```python
from build123d import *

# Parameters (mm, degrees)
SKETCH1_W           = 82.539998569
SKETCH1_H           = 65.04
BOSS_EXTRUDE1_DEPTH = 43.18
SHELL1_T            = 2.54
CUT_EXTRUDE2_DEPTH  = 124.028758627
SKETCH7_W           = 87.619998569
SKETCH7_H           = 43.18
BOSS_EXTRUDE2_DEPTH = 2.54
CUT_EXTRUDE3_DEPTH  = 2.54
CUT_EXTRUDE4_DEPTH  = 2.54
SKETCH10_W          = 1.27
SKETCH10_H          = 35.56
CUT_EXTRUDE5_DEPTH  = 2.54
SKETCH11_W          = 12.7
SKETCH11_H          = 2.54
BOSS_EXTRUDE3_DEPTH = 12.7
CUT_EXTRUDE7_DEPTH  = 125.717897357
SKETCH13_W          = 12.7
SKETCH13_H          = 12.7
SKETCH13_R          = 2.1
BOSS_EXTRUDE4_DEPTH = 3.175
FILLET2_R           = 3


with BuildPart() as part:
    # Sketch1 → Boss-Extrude1 (new body)
    with BuildSketch(Plane.XY):
        with Locations((47.599999189, 40.75)):
            Rectangle(SKETCH1_W, SKETCH1_H)
    extrude(amount=BOSS_EXTRUDE1_DEPTH)

    # Shell1
    shell1_openings = [part.faces().sort_by_distance(p)[0] for p in [
        (47.599999189, 73.27, 21.59),
        (47.599999189, 40.75, 0),
    ]]
    offset(amount=SHELL1_T, openings=shell1_openings, kind=Kind.INTERSECTION)

    # Sketch6 → Cut-Extrude2 (cut, through all)
    with BuildSketch(Plane.ZY.offset(-3.789999905)):
        Polygon((2.54, 59.03), (2.54, 73.27), (0, 73.27), (0, 59.03), (0, 3.15), (38.1, 3.15), (38.1, 19.92924), (2.54, 19.92924), align=None)
    extrude(amount=-CUT_EXTRUDE2_DEPTH, mode=Mode.SUBTRACT)

    # Sketch7 → Boss-Extrude2 (add)
    with BuildSketch(Plane(origin=(0, 73.27, 0), x_dir=(1, 0, 0), z_dir=(0, 1, 0))):
        with Locations((47.59999919, -24.13)):
            Rectangle(SKETCH7_W, SKETCH7_H)
    extrude(amount=BOSS_EXTRUDE2_DEPTH)

    # Sketch8 → Cut-Extrude3 (cut)
    with BuildSketch(Plane(origin=(0, 0, 2.54), x_dir=(-1, 0, 0), z_dir=(0, 0, -1))):
        Polygon((-65.405564728, 73.27), (-65.405564728, 74.54), (-90.139998474, 74.54), (-90.139998474, 19.92924), (-88.869998474, 19.92924), (-88.869998474, 73.27), align=None)
        Polygon((-5.059999905, 74.54), (-65.405564728, 74.54), (-65.405564728, 73.27), (-6.329999905, 73.27), (-6.329999905, 19.92924), (-5.059999905, 19.92924), align=None)
    extrude(amount=-CUT_EXTRUDE3_DEPTH, mode=Mode.SUBTRACT)

    # Sketch9 → Cut-Extrude4 (cut)
    with BuildSketch(Plane(origin=(0, 0, 38.1), x_dir=(-1, 0, 0), z_dir=(0, 0, -1))):
        Polygon((-90.139998474, 19.92924), (-90.139998474, 6.96), (-5.059999905, 6.96), (-5.059999905, 19.92924), (-6.329999905, 19.92924), (-6.329999905, 8.23), (-88.869998474, 8.23), (-88.869998474, 19.92924), align=None)
    extrude(amount=-CUT_EXTRUDE4_DEPTH, mode=Mode.SUBTRACT)

    # Sketch10 → Cut-Extrude5 (cut)
    with BuildSketch(Plane.XZ.offset(-19.92924)):
        with Locations((5.694999905, 22.86)):
            Rectangle(SKETCH10_W, SKETCH10_H)
        with Locations((89.504998474, 22.86)):
            Rectangle(SKETCH10_W, SKETCH10_H)
    extrude(amount=-CUT_EXTRUDE5_DEPTH, mode=Mode.SUBTRACT)

    # Sketch11 → Boss-Extrude3 (add)
    with BuildSketch(Plane.XZ.offset(-5.69)):
        with Locations((11.409999905, 39.37)):
            Rectangle(SKETCH11_W, SKETCH11_H)
        with Locations((83.789998474, 39.37)):
            Rectangle(SKETCH11_W, SKETCH11_H)
    extrude(amount=BOSS_EXTRUDE3_DEPTH)

    # Sketch12 → Cut-Extrude7 (cut, through all)
    with BuildSketch(Plane.XY.offset(40.64)):
        with BuildLine():
            Line((9.309999905, 0.61), (9.309999905, -1.683510845))
            ThreePointArc((9.309999905, -1.683510845), (11.409999905, -3.783510845), (13.509999905, -1.683510845))
            Line((13.509999905, -1.683510845), (13.509999905, 0.61))
            ThreePointArc((13.509999905, 0.61), (11.409999905, 2.71), (9.309999905, 0.61))
        make_face()
        with BuildLine():
            Line((81.689998474, 0.61), (81.689998474, -1.683510845))
            ThreePointArc((81.689998474, -1.683510845), (83.789998474, -3.783510845), (85.889998474, -1.683510845))
            Line((85.889998474, -1.683510845), (85.889998474, 0.61))
            ThreePointArc((85.889998474, 0.61), (83.789998474, 2.71), (81.689998474, 0.61))
        make_face()
    extrude(amount=-CUT_EXTRUDE7_DEPTH, mode=Mode.SUBTRACT)

    # Sketch13 → Boss-Extrude4 (add)
    # profile 1 of 2: a face of its own
    with BuildSketch(Plane(origin=(0, 0, 2.54), x_dir=(-1, 0, 0), z_dir=(0, 0, -1))):
        with Locations((-97.759998474, 69.46)):
            Rectangle(SKETCH13_W, SKETCH13_H)
        with Locations((-97.759998474, 69.46)):
            Circle(SKETCH13_R, mode=Mode.SUBTRACT)
    # profile 2 of 2: a face of its own
    with BuildSketch(Plane(origin=(0, 0, 2.54), x_dir=(-1, 0, 0), z_dir=(0, 0, -1))):
        with Locations((2.560000095, 69.46)):
            Rectangle(SKETCH13_W, SKETCH13_H)
        with Locations((2.560000095, 69.46)):
            Circle(SKETCH13_R, mode=Mode.SUBTRACT)
    extrude(amount=-BOSS_EXTRUDE4_DEPTH)

    # Fillet2
    fillet2_edges = [part.edges().sort_by_distance(p)[0] for p in [
        (17.759999905, 5.69, 39.37),
        (5.059999905, -7.01, 39.37),
        (17.759999905, -7.01, 39.37),
        (77.439998474, 5.69, 39.37),
        (90.139998474, -7.01, 39.37),
        (77.439998474, -7.01, 39.37),
        (91.409998474, 63.11, 4.1275),
        (104.109998474, 63.11, 4.1275),
        (104.109998474, 75.81, 4.1275),
        (3.789999905, 75.81, 25.7175),
        (3.789999905, 63.11, 4.1275),
        (-8.910000095, 75.81, 4.1275),
        (-8.910000095, 63.11, 4.1275),
        (91.409998474, 75.81, 25.7175),
        (91.409998474, 5.69, 41.91),
        (3.789999905, 5.69, 41.91),
    ]]
    fillet(fillet2_edges, radius=FILLET2_R)


solid = part.part
```
The listing builds one solid part. Answer for the finished solid, in the listing's coordinates (mm). A direction names the side the tool comes from. Give positions to 0.01 mm unless a question says otherwise; leave off trailing zeros. Loops run counter-clockwise (first coordinate to the right, second up) from the corner with the lowest first, then second, coordinate; pieces in that order, holes last. Notation, with made-up numbers: M 28.5,2.5 L 54.5,2.5 A28 cw 54.5,41.5 Z; hole C 0.25,24 d10. An arc over 180 degrees is marked long. One line per item, written item: value.
Q1. A cutting plane is placed at D-D on x = 63. Determine the outline of the cut face in (y, z), then the cut area to 3 significant figures.
Working result:
outline: M 5.69,38.1 L 6.96,38.1 L 6.96,40.64 L 8.23,40.64 L 8.23,43.18 L 73.27,43.18 L 73.27,5.08 L 74.54,5.08 L 74.54,2.54 L 75.81,2.54 L 75.81,45.72 L 5.69,45.72 Z
area: 288 mm^2
Q2. For faces 1 (the face through (98, 63.11, 4)), 2 (the face through (47.4, 7.2, 40.64)), 3 (the face through (48, 74, 5.08)), 4 (the face through (51, 6, 38.1)), 5 (the face through (16.9, -6.11, 39.39)), determine the directions among +Z, -Z, +X, -X, +Y, -Y from which every point of the face is accessible in a straight line to the end or side of a thin tool.
Working result:
face 1: +Z, -Z, +X, -Y
face 2: -Z
face 3: -Z, -Y
face 4: -Z, +X, -X, -Y
face 5: +Z, -Z, -Y
Q3. A cutting plane is placed at B-B on x = 11.41. Determine the outline of the cut face in (y, z), then the cut area to 3 significant figures.
Working result:
outline: M -7.01,38.1 L -3.78,38.1 L -3.78,40.64 L -7.01,40.64 Z; M 2.71,38.1 L 6.96,38.1 L 6.96,40.64 L 8.23,40.64 L 8.23,43.18 L 73.27,43.18 L 73.27,5.08 L 74.54,5.08 L 74.54,2.54 L 75.81,2.54 L 75.81,45.72 L 5.69,45.72 L 5.69,40.64 L 2.71,40.64 Z
area: 304 mm^2
Q4. Flat-ended cylindrical pins translate along their axes: P1, Ø1.4, axis at x = 6, z = 27.5, coming from the -Y side; P2, Ø5, axis at x = 97.76, y = 69.46, coming from the +Z side (3 decimals); P3, Ø1.5, axis at y = 37, z = 14, coming from the -X side. Find the tip coordinate at first contact, or state that the pin passes through.
Working result:
P1: stops at y = 22.47
P2: stops at z = 5.715
P3: stops at x = 3.79
Q5. A cutting plane is placed at C-C on z = 18. Determine the outline of the cut face in (x, y).
Working result:
outline: M 3.79,19.93 L 5.06,19.93 L 5.06,22.47 L 6.33,22.47 L 6.33,73.27 L 88.87,73.27 L 88.87,22.47 L 90.14,22.47 L 90.14,19.93 L 91.41,19.93 L 91.41,72.81 A3 ccw 88.41,75.81 L 6.79,75.81 A3 ccw 3.79,72.81 Z
Q6. Find the intervals of material crossed by line 1 (Y direction, x = -2.56, z = 3.95); line 2 (X direction, y = 22, z = 33); line 3 (Y direction, x = 32, z = 40), in increasing order. Write a range as from..to.
Working result:
line 1: y = 63.11..67.36, 71.56..75.81
line 2: x = 3.79..5.06, 90.14..91.41
line 3: y = 5.69..6.96, 73.27..75.81
Q7. A cutting plane is placed at A-A on y = 69.46. Determine the outline of the cut face in (x, z) (3 decimals).
Working result:
outline: M -8.91,2.54 L -4.66,2.54 L -4.66,5.715 L -8.91,5.715 Z; M -0.46,2.54 L 5.06,2.54 L 5.06,5.08 L 6.33,5.08 L 6.33,43.18 L 88.87,43.18 L 88.87,5.08 L 90.14,5.08 L 90.14,2.54 L 95.66,2.54 L 95.66,5.715 L 91.41,5.715 L 91.41,45.72 L 3.79,45.72 L 3.79,5.715 L -0.46,5.715 Z; M 99.86,2.54 L 104.11,2.54 L 104.11,5.715 L 99.86,5.715 Z
